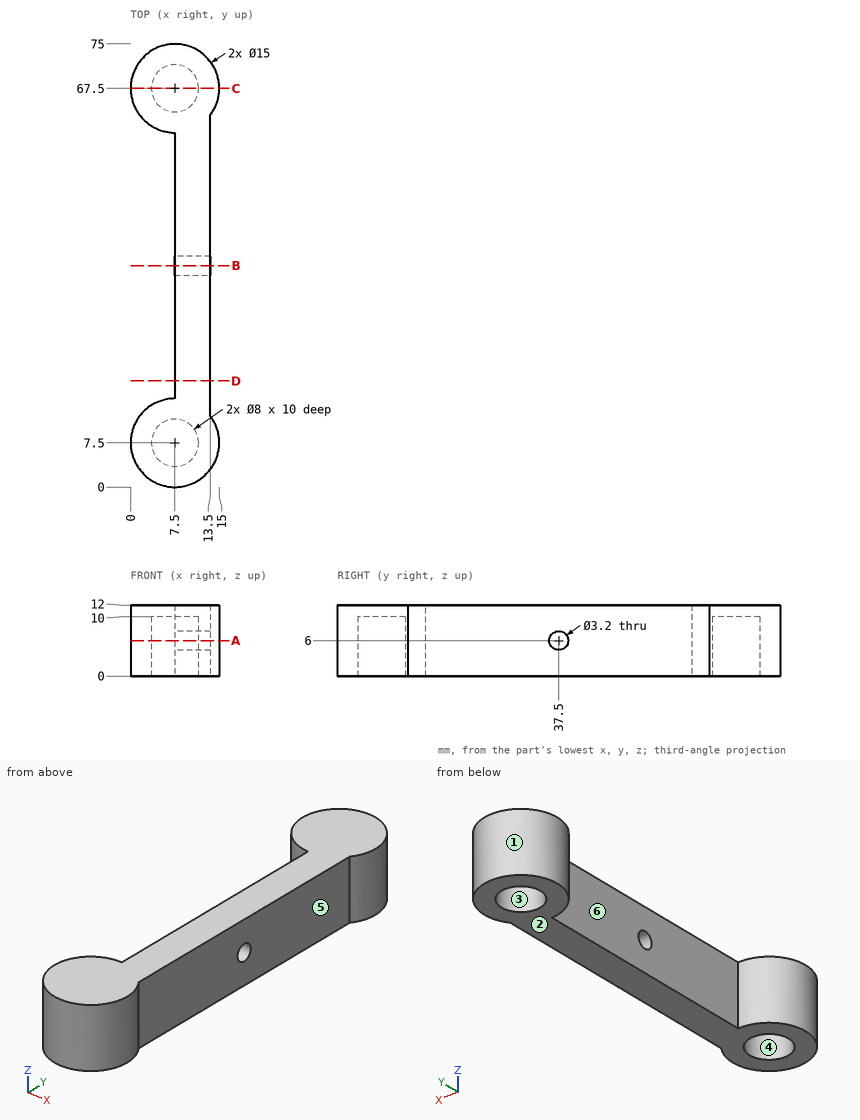
The figure shows three views and two pictorial views of one solid part (mm, origin at its lowest corner). Answer the questions. A direction names the side the tool comes from. Round coordinates to 2 decimals unless told otherwise and drop trailing zeros. Write each loop counter-clockwise with the first axis right and the second up, starting at its lowest first coordinate (ties: lowest second). Pieces come first, ordered by that corner, then holes. Notation, with made-up numbers: (14, 37) - (47, 37) arc R18 cw to (47, 52) - close; hole circle Ø11 at (-15.5, 23.5). An arc over 180 degrees is marked (long way). Answer in a Markdown table with one row per item. Add a question column.
1. A cutting plane is placed at B-B, the plane y = 37.5. Determine the outline of the cut face in (x, z), and give its area (3 significant figures).
2. A cutting plane is placed at C-C, the plane y = 67.5. Determine the outline of the cut face in (x, z).
3. A cutting plane is placed at D-D, the plane y = 18. Determine the outline of the cut face in (x, z).
4. The mould has two halves that part along X. Classify the marked faces 1, 2 and 3: +X half, -X half, draft (parallel to the pull), parting line (faces both ways), or undercut.
5. For the marked faces 4, 5 and 6, determine the directions among +Z, -Z, +X, -X, +Y, -Y from which every point of the face is accessible in a straight line to the end or side of a thin tool.
6. A cutting plane is placed at A-A, the plane z = 6. Determine the outline of the cut face in (x, y), and give its area (3 significant figures).
7. Find the intervals of material crossed by line 1 along Z through (x, y) = (11.3, 37.5); line 2 along Y through (x, z) = (5.5, 5); line 3 along Y through (x, z) = (7.75, 3), in increasing order. Write a range as from..to.
8. Given pin 1 (4 mm diameter, centred on y = 37.5, z = 6, fed in from -X); pin 2 (6.5 mm diameter, centred on x = 7.5, y = 67.5, fed in from -Z); pin 3 (3 mm diameter, centred on x = 13, z = 9.5, fed in from +Y), each flat-ended and moving along its own axis, determine where each tip first touches the part or whether it passes through.
Worked out:
| question | item | result |
|---|---|---|
| 1 | outline | (7.5, 0) - (13.5, 0) - (13.5, 4.4) - (7.5, 4.4) - close; (7.5, 7.6) - (13.5, 7.6) - (13.5, 12) - (7.5, 12) - close |
| 1 | area | 52.8 mm^2 |
| 2 | outline | (0, 0) - (3.5, 0) - (3.5, 10) - (11.5, 10) - (11.5, 0) - (15, 0) - (15, 12) - (0, 12) - close |
| 3 | outline | (7.5, 0) - (13.5, 0) - (13.5, 12) - (7.5, 12) - close |
| 4 | face 1 | parting line |
| 4 | face 2 | draft |
| 4 | face 3 | undercut |
| 5 | face 4 | -Z |
| 5 | face 5 | +Z, -Z, +X |
| 5 | face 6 | +Z, -Z, -X |
| 6 | outline | (7.5, 15) arc R7.5 ccw (long way) to (13.5, 12) - (13.5, 35.9) - (7.5, 35.9) - close; (7.5, 39.1) - (13.5, 39.1) - (13.5, 63) arc R7.5 ccw (long way) to (7.5, 60) - close; hole circle Ø8 at (7.5, 7.5); hole circle Ø8 at (7.5, 67.5) |
| 6 | area | 515 mm^2 |
| 7 | line 1 | 0..4.4, 7.6..12 |
| 7 | line 2 | 0.27..4.04, 10.96..14.73, 60.27..64.04, 70.96..74.73 |
| 7 | line 3 | 0..3.51, 11.49..63.51, 71.49..75 |
| 8 | pin 1 | x = 7.5 |
| 8 | pin 2 | z = 10 |
| 8 | pin 3 | y = 73.84 |
